Can you work these out from the drawing? Everything is in mm from the part's minimum corner. A direction names the side the tool comes from. Coordinates: 2 decimals unless noted, no trailing zeros. Loops run counter-clockwise (first coordinate to the right, second up) from the corner with the lowest first, then second, coordinate; pieces in that order, holes last. Notation, with made-up numbers: M -4,25.25 L 19,25.25 A20 ccw 19,60.25 Z; hole C 1.25,73.5 d9. An arc over 180 degrees is marked long. Use CSV: the item, a comma, the result in double quotes. Start each with the question number.
Q1. Please list where this line runs through material, in increasing order: probe 1 along Y at (x, z) = (30.5, 7) (3 decimals). Write a range as [from, to].
Q2. For pin 1 Ø2 at (x, z) = (70, 16.5) entering from +Y (3 decimals); pin 2 Ø1.5 at (x, y) = (50, 10) entering from +Z (3 decimals), each with a flat end and sliding along its axis, tell me the tip position at first contact or that it passes through.
Q3. If we section it at B-B (y = 10): Please give me the cut outline in (x, z) (3 decimals).
Q4. If we section it at A-A (x = 131): Please give me the cut outline in (y, z) (3 decimals).
Q5. Which directions (+Z, -Z, +X, -X, +Y, -Y) give clear straight access to the entire face, cutting with the end or side of a thin tool? Please do the marked faces 1 and 2.
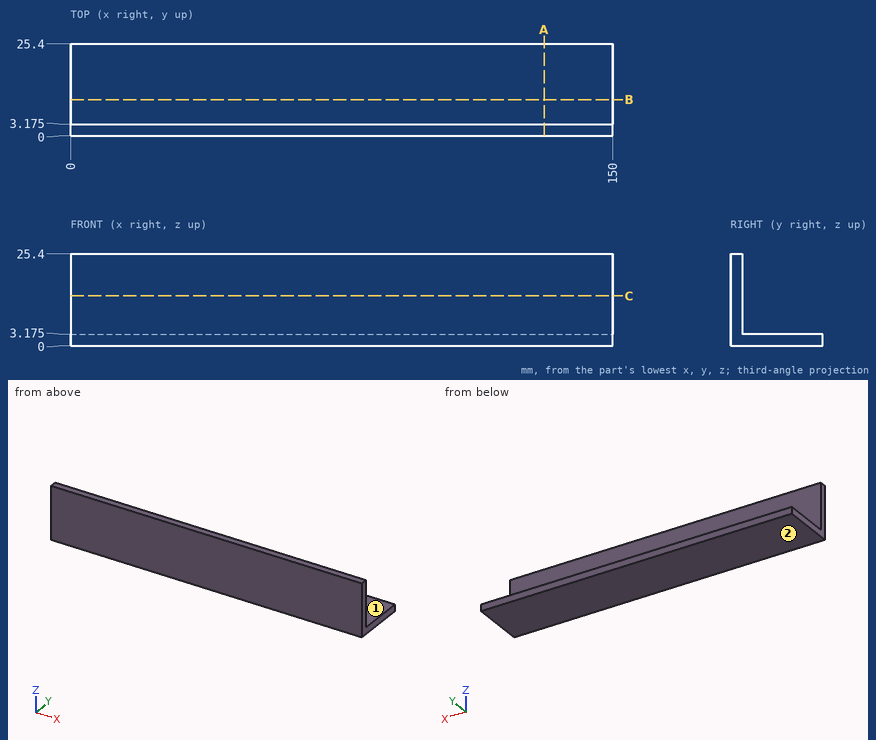
Results below:
1,probe 1,"[0, 3.175]"
2,pin 1,"y = 3.175"
2,pin 2,"z = 3.175"
3,outline,"M 0,0 L 150,0 L 150,3.175 L 0,3.175 Z"
4,outline,"M 0,0 L 25.4,0 L 25.4,3.175 L 3.175,3.175 L 3.175,25.4 L 0,25.4 Z"
5,face 1,"+Z, +X, -X, +Y"
5,face 2,"-Z, +X, -X, +Y, -Y"
